from build123d import *

# Parameters (mm, degrees)
SKETCH1_R              = 9.525
BOSS_EXTRUDE1_DEPTH    = 3
CUT_EXTRUDE1_DEPTH     = 72.404901793
SKETCH4_W              = 50.8
SKETCH4_H              = 19.4
BOSS_EXTRUDE3_DEPTH    = 6
SKETCH3_W              = 6
SKETCH3_H              = 12.7
BOSS_EXTRUDE2_DEPTH    = 6
FILLET1_R              = 1.5875
LPATTERN1_COUNT        = 5
LPATTERN1_PITCH        = 25.4
FILLET1_OF_LPATTERN1_R = 1.5875
SKETCH5_W              = 12.7
SKETCH5_H              = 6
BOSS_EXTRUDE4_DEPTH    = 6
FILLET2_R              = 1.5875
LPATTERN2_COUNT        = 2
LPATTERN2_PITCH        = 25.4
FILLET2_OF_LPATTERN2_R = 1.5875
CUT_EXTRUDE2_DEPTH     = 121.632085284
FILLET3_R              = 2.54


with BuildPart() as part:
    # Sketch1 → Boss-Extrude1 (new, symmetric)
    with BuildSketch(Plane(origin=(0, 0, 0), x_dir=(0, 0, -1), z_dir=(1, 0, 0))):
        with BuildLine():
            Line((-15.540953853, 3.23950279), (-9.525, 32.1))
            Line((-9.525, 32.1), (63.5, 32.1))
            Line((63.5, 32.1), (63.5, -15.875))
            Line((63.5, -15.875), (0, -15.875))
            ThreePointArc((0, -15.875), (-12.317522717, -10.014702148), (-15.540953853, 3.23950279))
        make_face()
        Circle(SKETCH1_R, mode=Mode.SUBTRACT)
    extrude(amount=BOSS_EXTRUDE1_DEPTH, both=True)

    # Sketch2 → Cut-Extrude1 (cut, through all)
    with BuildSketch(Plane(origin=(3, 0, 0), x_dir=(0, 0, -1), z_dir=(1, 0, 0))):
        with BuildLine():
            Line((6.834450038, -14.328500189), (63.5, 12.7))
            Line((63.5, 12.7), (63.5, -15.875))
            Line((63.5, -15.875), (0, -15.875))
            ThreePointArc((0, -15.875), (3.50361845, -15.483548778), (6.834450038, -14.328500189))
        make_face()
    extrude(amount=-CUT_EXTRUDE1_DEPTH, mode=Mode.SUBTRACT)

    # Sketch4 → Boss-Extrude3 (add)
    with BuildSketch(Plane(origin=(3, 0, 0), x_dir=(0, 0, -1), z_dir=(1, 0, 0))):
        with Locations((88.9, 22.4)):
            Rectangle(SKETCH4_W, SKETCH4_H)
    extrude(amount=-BOSS_EXTRUDE3_DEPTH)

    # Sketch3 → Boss-Extrude2 (add)
    with BuildSketch(Plane(origin=(0, 32.1, 0), x_dir=(1, 0, 0), z_dir=(0, 1, 0))):
        Rectangle(SKETCH3_W, SKETCH3_H)
    boss_extrude2 = extrude(amount=BOSS_EXTRUDE2_DEPTH)

    # Fillet1
    fillet1_edges = [part.edges().sort_by_distance(p)[0] for p in [
        (0, 38.1, -6.35),
        (0, 38.1, 6.35),
    ]]
    fillet(fillet1_edges, radius=FILLET1_R)

    # LPattern1: Boss-Extrude2 ×5
    with Locations(*[(0, 0, -i * LPATTERN1_PITCH) for i in range(1, LPATTERN1_COUNT)]):
        add(boss_extrude2)

    # Fillet1 of LPattern1
    fillet1_of_lpattern1_edges = [part.edges().sort_by_distance(p)[0] for p in [
        (0, 38.1, -31.75),
        (0, 38.1, -19.05),
        (0, 38.1, -57.15),
        (0, 38.1, -44.45),
        (0, 38.1, -82.55),
        (0, 38.1, -69.85),
        (0, 38.1, -107.95),
        (0, 38.1, -95.25),
    ]]
    fillet(fillet1_of_lpattern1_edges, radius=FILLET1_OF_LPATTERN1_R)

    # Sketch5 → Boss-Extrude4 (add)
    with BuildSketch(Plane.ZY.offset(3)):
        with Locations((-76.2, 9.7)):
            Rectangle(SKETCH5_W, SKETCH5_H)
    boss_extrude4 = extrude(amount=-BOSS_EXTRUDE4_DEPTH)

    # Fillet2
    fillet2_edges = [part.edges().sort_by_distance(p)[0] for p in [
        (0, 6.7, -82.55),
        (0, 6.7, -69.85),
    ]]
    fillet(fillet2_edges, radius=FILLET2_R)

    # LPattern2: Boss-Extrude4 ×2
    with Locations(*[(0, 0, -i * LPATTERN2_PITCH) for i in range(1, LPATTERN2_COUNT)]):
        add(boss_extrude4)

    # Fillet2 of LPattern2
    fillet2_of_lpattern2_edges = [part.edges().sort_by_distance(p)[0] for p in [
        (0, 6.7, -107.95),
        (0, 6.7, -95.25),
    ]]
    fillet(fillet2_of_lpattern2_edges, radius=FILLET2_OF_LPATTERN2_R)

    # Sketch6 → Cut-Extrude2 (cut, through all)
    with BuildSketch(Plane(origin=(3, 0, 0), x_dir=(0, 0, -1), z_dir=(1, 0, 0))):
        with BuildLine():
            Line((-1.27, 27.02), (-5.394730621, 27.02))
            Line((-5.394730621, 27.02), (-8.560402164, 11.83323877))
            ThreePointArc((-8.560402164, 11.83323877), (-0.341722831, 14.601001695), (7.997440758, 12.220759646))
            Line((7.997440758, 12.220759646), (21.902982951, 27.02))
            Line((21.902982951, 27.02), (1.27, 27.02))
            Line((1.27, 27.02), (-1.27, 27.02))
        make_face()
        with BuildLine():
            ThreePointArc((14.605, 0), (14.332832255, -2.806411331), (13.526472843, -5.50822634))
            Line((13.526472843, -5.50822634), (58.749014948, 16.062154405))
            Line((58.749014948, 16.062154405), (26.218568583, 24.19428546))
            Line((26.218568583, 24.19428546), (11.699586285, 8.742179692))
            ThreePointArc((11.699586285, 8.742179692), (13.859626306, 4.606168001), (14.605, 0))
        make_face()
    extrude(amount=-CUT_EXTRUDE2_DEPTH, mode=Mode.SUBTRACT)

    # Fillet3
    fillet3_edges = [part.edges().sort_by_distance(p)[0] for p in [
        (0, -5.50822634, -13.526472843),
        (0, 8.742179692, -11.699586285),
        (0, 24.19428546, -26.218568583),
        (0, 16.062154405, -58.749014948),
        (0, 12.220759646, -7.997440758),
        (0, 11.83323877, 8.560402164),
        (0, 27.02, 5.394730621),
        (0, 27.02, -21.902982951),
    ]]
    fillet(fillet3_edges, radius=FILLET3_R)


solid = part.part
Can you work these out from the model? Positions are in its coordinate system, mm. A direction names the side the tool comes from. Round coordinates to 2 decimals unless told otherwise and drop trailing zeros. Loops run counter-clockwise (first coordinate to the right, second up) from the corner with the lowest first, then second, coordinate; pieces in that order, holes last. Notation, with made-up numbers: (69, 78) - (98, 78) arc R16 cw to (98, 99) - close; hole circle Ø6 at (64.5, 69). An arc over 180 degrees is marked (long way). Write item = value, one per line. Start each with the question number.
(1) If we section it at A-A (z = -50.5): Please give me the cut outline in (x, y), and give its area (3 significant figures).
(2) If we section it at C-C (x = -0.75): Give the number of separate pieces and of enclosed holes in the cut face, and give its area (3 significant figures).
(3) If we section it at B-B (z = -92): Please give me the cut outline in (x, y).
(4) For P1, Ø2, axis at x = -1, y = 35.5, coming from the -Z side; P2, Ø3, axis at x = -1, z = -110.5, coming from the +Y side; P3, Ø1.3, axis at x = -1, y = 11, coming from the +Z side, each with a flat end and sliding along its axis, tell me the tip position at first contact or that it passes through.
(5) If I drill on probe 1 along Y at (x, z) = (-1.2, 0) (3 decimals); probe 2 along Y at (x, z) = (2.5, 3); probe 3 along Y at (x, z) = (-0.5, -94), over which ranges is the centre line in solid material (lowest first)? Write a range as [from, to].
(6) If we mould it in two halves opening along Z, with no side actions, what happens to faces 1 (the face through (0, 32.1, -111)), 2 (the face through (0, 10, -107.95)), 3 (the face through (-0.04, 14.54, 6.75))? For each: released by +Z, released by -Z, zero draft, split by the parting line, or undercut.
(7) For faces 4 (the face through (0, 8.8, -12.4)), 5 (the face through (0, 34, -82.55)), 6 (the face through (0, 34, 6.35)), 7 (the face through (0, 12.7, -89)), which set-ups out of +Z, -Z, +X, -X, +Y, -Y let a thin tool reach every point of the face, with its end or its side?
Ans:
q1.outline = (-3, 6.5) - (3, 6.5) - (3, 12.13) - (-3, 12.13) - close; (-3, 18.12) - (3, 18.12) - (3, 38.1) - (-3, 38.1) - close
q1.area = 154 mm²
q2.separate_pieces = 1
q2.enclosed_holes = 3
q2.area = 3,130 mm²
q3.outline = (-3, 12.7) - (3, 12.7) - (3, 32.1) - (-3, 32.1) - close
q4.P1 = -107.95
q4.P2 = 32.1
q4.P3 = 14.06
q5.probe_1 = [-15.875, -9.525], [9.525, 14.605], [27.02, 38.1]
q5.probe_2 = [-15.59, -9.04], [9.04, 14.29], [27.02, 38.1]
q5.probe_3 = [12.7, 32.1]
q6.face_1 = zero draft
q6.face_2 = released by -Z
q6.face_3 = undercut
q7.face_4 = +X, -X
q7.face_5 = +X, -X, +Y
q7.face_6 = +Z, +X, -X, +Y
q7.face_7 = +X, -X, -Y
